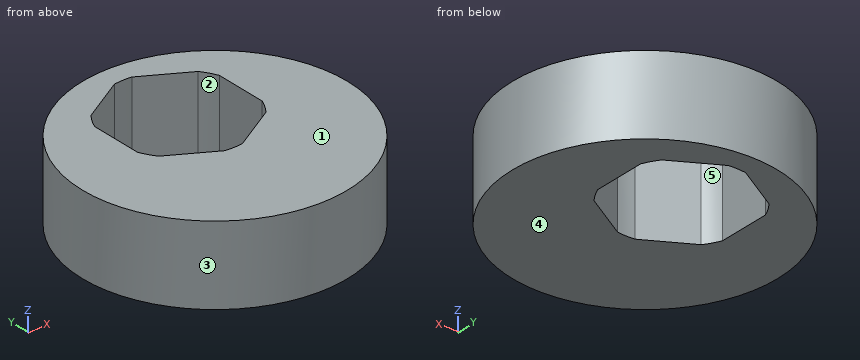
from build123d import *

# Parameters (mm, degrees)
SKETCH1_R           = 13.5
BOSS_EXTRUDE1_DEPTH = 4
CUT_EXTRUDE1_DEPTH  = 21.700241544


with BuildPart() as part:
    # Sketch1 → Boss-Extrude1 (new, symmetric)
    with BuildSketch(Plane.XY):
        Circle(SKETCH1_R)
    extrude(amount=BOSS_EXTRUDE1_DEPTH, both=True)

    # Sketch2 → Cut-Extrude1 (cut, through all)
    with BuildSketch(Plane.XY.offset(4)):
        with BuildLine():
            Line((-0.893039494, 11.316751826), (-5.456960506, 8.681770802))
            ThreePointArc((-5.456960506, 8.681770802), (-5.953924651, 7.9375), (-6.35, 7.134981025))
            Line((-6.35, 7.134981025), (-6.35, 1.865018975))
            ThreePointArc((-6.35, 1.865018975), (-5.953924651, 1.0625), (-5.456960506, 0.318229198))
            Line((-5.456960506, 0.318229198), (-0.893039494, -2.316751826))
            ThreePointArc((-0.893039494, -2.316751826), (0, -2.375), (0.893039494, -2.316751826))
            Line((0.893039494, -2.316751826), (5.456960506, 0.318229198))
            ThreePointArc((5.456960506, 0.318229198), (5.953924651, 1.0625), (6.35, 1.865018975))
            Line((6.35, 1.865018975), (6.35, 7.134981025))
            ThreePointArc((6.35, 7.134981025), (5.953924651, 7.9375), (5.456960506, 8.681770802))
            Line((5.456960506, 8.681770802), (0.893039494, 11.316751826))
            ThreePointArc((0.893039494, 11.316751826), (0, 11.375), (-0.893039494, 11.316751826))
        make_face()
    extrude(amount=-CUT_EXTRUDE1_DEPTH, mode=Mode.SUBTRACT)


solid = part.part
Work out the finished part from the listing and answer in its coordinate system (mm). Face numbers are marked on the shaded views. A direction names the side the tool comes from. Coordinates: 2 decimals unless noted, no trailing zeros. Write each loop counter-clockwise with the first axis right and the second up, starting at its lowest first coordinate (ties: lowest second). Pieces come first, ordered by that corner, then holes. Notation, with made-up numbers: M -39,15 L 15,15 A29 cw 15,42 Z; hole C 10.25,89 d2. An arc over 180 degrees is marked long. Answer as CSV lines item,"result". Start each with the question number.
Item 1: Section C-C on z = -1 is taken. Write down the section's boundary in (x, y) (3 decimals), and give its area (3 significant figures).
Item 2: Consider L1, parallel to Y at x = 0, z = 2.25 (3 decimals); L2, parallel to X at y = -0.5, z = -3.25; L3, parallel to Y at x = 3.5, z = -0.5. Determine where each line is inside the solid, lowest interval first.
Item 3: Section B-B on y = 9.25 is taken. Write down the section's boundary in (x, z), and give its area (3 significant figures).
Item 4: Determine the mould class of the marked faces 1, 2 and 3 for opening direction Y: released by +Y, released by -Y, zero draft, split by the parting line, or undercut.
Item 5: Section D-D on y = -6.75 is taken. Write down the section's boundary in (x, z).
Item 6: Section A-A on x = 0 is taken. Write down the section's boundary in (y, z) (3 decimals), and give its area (3 significant figures).
Item 7: A tool of negligible diameter and unlimited length cuts with its end or side. For the marked faces 4 and 5, from which of +Z, -Z, +X, -X, +Y, -Y can it reach the whole face along a straight path? Write none if from no direction.
Item 8: Flat-ended cylindrical pins translate along their axes: P1, Ø2.5, axis at y = 4, z = -0.5, coming from the -X side; P2, Ø1, axis at x = -6.5, z = 3, coming from the +Y side; P3, Ø3, axis at y = -4.5, z = -0.5, coming from the +X side. Find the tip coordinate at first contact, or state that the pin passes through.
Checks:
1,outline,"C 0,0 d27; hole M -6.35,1.865 A6.875 ccw -5.457,0.318 L -0.893,-2.317 A6.875 ccw 0.893,-2.317 L 5.457,0.318 A6.875 ccw 6.35,1.865 L 6.35,7.135 A6.875 ccw 5.457,8.682 L 0.893,11.317 A6.875 ccw -0.893,11.317 L -5.457,8.682 A6.875 ccw -6.35,7.135 Z"
1,area,"435 mm²"
2,L1,"y = -13.5 to -2.375, 11.375 to 13.5"
2,L2,"x = -13.49 to -4.04, 4.04 to 13.49"
2,L3,"y = -13.04 to -0.81, 9.81 to 13.04"
3,outline,"M -9.83,-4 L -4.47,-4 L -4.47,4 L -9.83,4 Z; M 4.47,-4 L 9.83,-4 L 9.83,4 L 4.47,4 Z"
3,area,"85.8 mm²"
4,face 1,"zero draft"
4,face 2,"undercut"
4,face 3,"split by the parting line"
5,outline,"M -11.69,-4 L 11.69,-4 L 11.69,4 L -11.69,4 Z"
6,outline,"M -13.5,-4 L -2.375,-4 L -2.375,4 L -13.5,4 Z; M 11.375,-4 L 13.5,-4 L 13.5,4 L 11.375,4 Z"
6,area,"106 mm²"
7,face 4,"-Z, +X, -X, +Y, -Y"
7,face 5,"+Z, -Z"
8,P1,"stops at x = -13.22"
8,P2,"stops at y = 12.09"
8,P3,"stops at x = 13.16"
